Geometry: final body of the model. Coordinates: model frame, mm. A direction names the side the tool comes from. Round coordinates to 2 decimals unless told otherwise and drop trailing zeros. Order: outer loops, then holes, each group sorted by start corner. A loop starts at its lowest first (then second) coordinate and runs counter-clockwise, first axis right, second up. Notation, with made-up numbers: (-38.75, 40) -> (-28.75, 40) arc R31 cw to (-28.75, 66) -> close; hole circle Ø11 at (38, 20). An arc over 180 degrees is marked (long way). Put each result on its own line as item: value.
```python
from build123d import *

# Parameters (mm, degrees)
SALIENTE_EXTRUIR1_DEPTH = 6
CROQUIS2_R              = 3.9
SALIENTE_EXTRUIR2_DEPTH = 5.4
CHAFL_N1_SIZE           = 1
REDONDEO1_R             = 0.6
CHAFL_N2_SIZE           = 1


with BuildPart() as part:
    # Croquis1 → Saliente-Extruir1 (new body)
    with BuildSketch(Plane(origin=(0, 0, 0), x_dir=(0, 1, 0), z_dir=(0, 0, 1))):
        Polygon((5.8, -2.402438662), (5.8, 2.402438662), (2.402438662, 5.8), (-2.402438662, 5.8), (-5.8, 2.402438662), (-5.8, -2.402438662), (-2.402438662, -5.8), (2.402438662, -5.8), align=None)
    extrude(amount=SALIENTE_EXTRUIR1_DEPTH)

    # Croquis2 → Saliente-Extruir2 (add)
    with BuildSketch(Plane.XY.offset(6)):
        with Locations(Location((0, 0, 0), (0, 0, 180))):
            Circle(CROQUIS2_R)
    extrude(amount=SALIENTE_EXTRUIR2_DEPTH)

    # Chaflán1
    chafl_n1_edges = [part.edges().sort_by_distance(p)[0] for p in [
        (3.9, 0, 11.4),
    ]]
    chamfer(chafl_n1_edges, length=CHAFL_N1_SIZE)

    # Redondeo1
    redondeo1_edges = [part.edges().sort_by_distance(p)[0] for p in [
        (3.9, 0, 6),
    ]]
    fillet(redondeo1_edges, radius=REDONDEO1_R)

    # Chaflán2
    chafl_n2_edges = [part.edges().sort_by_distance(p)[0] for p in [
        (-5.8, 0, 0),
        (-4.101219331, 4.101219331, 0),
        (0, 5.8, 0),
        (4.101219331, 4.101219331, 0),
        (5.8, 0, 0),
        (4.101219331, -4.101219331, 0),
        (0, -5.8, 0),
        (-4.101219331, -4.101219331, 0),
    ]]
    chamfer(chafl_n2_edges, length=CHAFL_N2_SIZE)


solid = part.part
```
1. Cut plane A-A on x = 0. Return loops of the section in (y, z).
Ans:
outline: (-5.8, 1) -> (-4.8, 0) -> (4.8, 0) -> (5.8, 1) -> (5.8, 6) -> (4.5, 6) arc R0.6 cw to (3.9, 6.6) -> (3.9, 10.4) -> (2.9, 11.4) -> (-2.9, 11.4) -> (-3.9, 10.4) -> (-3.9, 6.6) arc R0.6 cw to (-4.5, 6) -> (-5.8, 6) -> close
2. Cut plane C-C on z = 7.75. Return loops of the section in (x, y).
Ans:
outline: circle Ø7.8 at (0, 0)
3. Set-up query: faces 1 (the face through (-5.8, 0, 3)), 2 (the face through (2.87, -2.64, 8.47)). Return all of +Z, -Z, +X, -X, +Y, -Y with unobstructed straight access to the full face (end or side cutting, diameter ignored); none if empty.
Ans:
face 1: +Z, -Z, -X, +Y, -Y
face 2: +Z
4. Contact query for a flat-ended pin moving along its axis: P1, Ø1.5, axis at x = -4, z = 1.5, coming from the +Y side. Output: stop coordinate, or through.
Ans:
P1: y = 4.95
5. Material intervals for probe 1 along Z at (x, y) = (-3.75, 2.75); probe 2 along Y at (x, z) = (0.25, 6.5); probe 3 along Z at (x, y) = (3.25, -4), sorted ascending.
Ans:
probe 1: 0 to 6
probe 2: -3.9 to 3.9
probe 3: 0.33 to 6
6. Cut plane D-D on z = 6.25. Return loops of the section in (x, y).
Ans:
outline: circle Ø8.03 at (0, 0)
